Could you check a few things on this model? Use its own coordinates, in mm. Face numbers are marked on the shaded views. A direction names the side the tool comes from. Round coordinates to 2 decimals unless told otherwise and drop trailing zeros. Loops run counter-clockwise (first coordinate to the right, second up) from the corner with the lowest first, then second, coordinate; pieces in that order, holes last.
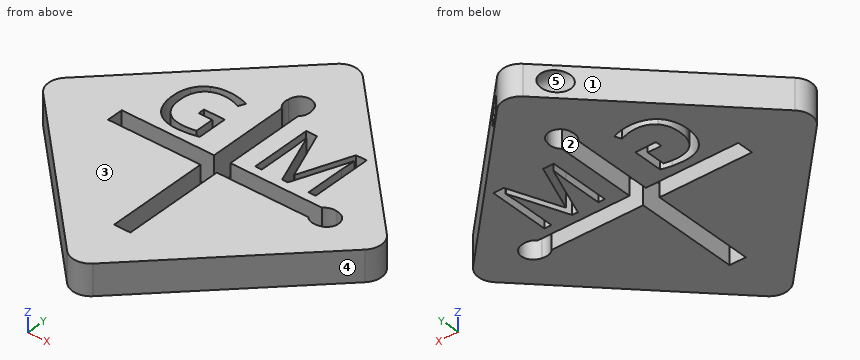
from build123d import *

# Parameters (mm, degrees)
F1_DEPTH = 2.5
F2_R     = 0.85
F3_DEPTH = 12.5


with BuildPart() as f1:
    # F0 (on Top) → F1 (new body)
    with BuildSketch(Plane.XY):
        with BuildLine():
            Line((13.081475452, -13.081475452), (1.0606601718, -1.0606601718))
            ThreePointArc((1.0606601718, -1.0606601718), (0, -0.6213203436), (-1.0606601718, -1.0606601718))
            Line((-1.0606601718, -1.0606601718), (-13.081475452, -13.081475452))
            ThreePointArc((-13.081475452, -13.081475452), (-13.5208152802, -14.1421356237), (-13.081475452, -15.2027957955))
            Line((-13.081475452, -15.2027957955), (-1.0606601718, -27.2236110757))
            ThreePointArc((-1.0606601718, -27.2236110757), (0, -27.6629509039), (1.0606601718, -27.2236110757))
            Line((1.0606601718, -27.2236110757), (13.081475452, -15.2027957955))
            ThreePointArc((13.081475452, -15.2027957955), (13.5208152802, -14.1421356237), (13.081475452, -13.081475452))
        make_face()
        with BuildLine():
            Line((-4.2551746457, -10.6432923429), (-4.2551746457, -10.1278843568))
            Line((-4.2551746457, -10.1278843568), (-2.5700617985, -10.1278843568))
            Line((-2.5700617985, -10.1278843568), (-2.5700617985, -12.5389086623))
            add(Edge.make_bspline(
                [(-2.5700617985, -12.5389086623), (-2.9639420069, -12.6647767179), (-3.3708430485, -12.7293383498)],
                knots=[0, 0, 0, 1, 1, 1], degree=2))
            add(Edge.make_bspline(
                [(-3.3708430485, -12.7293383498), (-3.7777440902, -12.7938999818), (-4.3137683957, -12.7938999818)],
                knots=[0, 0, 0, 1, 1, 1], degree=2))
            add(Edge.make_bspline(
                [(-4.3137683957, -12.7938999818), (-5.4389854096, -12.7938999818), (-6.0661555485, -12.1238695998)],
                knots=[0, 0, 0, 1, 1, 1], degree=2))
            add(Edge.make_bspline(
                [(-6.0661555485, -12.1238695998), (-6.6933256874, -11.4538392179), (-6.6933256874, -10.2472419957)],
                knots=[0, 0, 0, 1, 1, 1], degree=2))
            add(Edge.make_bspline(
                [(-6.6933256874, -10.2472419957), (-6.6933256874, -9.4735874818), (-6.3829958263, -8.8919902595)],
                knots=[0, 0, 0, 1, 1, 1], degree=2))
            add(Edge.make_bspline(
                [(-6.3829958263, -8.8919902595), (-6.0726659652, -8.3103930373), (-5.4894411388, -8.0038609193)],
                knots=[0, 0, 0, 1, 1, 1], degree=2))
            add(Edge.make_bspline(
                [(-5.4894411388, -8.0038609193), (-4.9062163124, -7.6973288012), (-4.123881243, -7.6973288012)],
                knots=[0, 0, 0, 1, 1, 1], degree=2))
            add(Edge.make_bspline(
                [(-4.123881243, -7.6973288012), (-3.3296104096, -7.6973288012), (-2.6449315902, -7.9881274123)],
                knots=[0, 0, 0, 1, 1, 1], degree=2))
            Line((-2.6449315902, -7.9881274123), (-2.8684558957, -8.4970249818))
            add(Edge.make_bspline(
                [(-2.8684558957, -8.4970249818), (-3.5401138819, -8.2127367873), (-4.1607736041, -8.2127367873)],
                knots=[0, 0, 0, 1, 1, 1], degree=2))
            add(Edge.make_bspline(
                [(-4.1607736041, -8.2127367873), (-5.0657215207, -8.2127367873), (-5.5746190902, -8.7514737665)],
                knots=[0, 0, 0, 1, 1, 1], degree=2))
            add(Edge.make_bspline(
                [(-5.5746190902, -8.7514737665), (-6.0835166596, -9.2902107457), (-6.0835166596, -10.2472419957)],
                knots=[0, 0, 0, 1, 1, 1], degree=2))
            add(Edge.make_bspline(
                [(-6.0835166596, -10.2472419957), (-6.0835166596, -11.2509312318), (-5.5936078055, -11.7695944262)],
                knots=[0, 0, 0, 1, 1, 1], degree=2))
            add(Edge.make_bspline(
                [(-5.5936078055, -11.7695944262), (-5.1036989513, -12.2882576207), (-4.1542631874, -12.2882576207)],
                knots=[0, 0, 0, 1, 1, 1], degree=2))
            add(Edge.make_bspline(
                [(-4.1542631874, -12.2882576207), (-3.6388552013, -12.2882576207), (-3.147318743, -12.1688999818)],
                knots=[0, 0, 0, 1, 1, 1], degree=2))
            Line((-3.147318743, -12.1688999818), (-3.147318743, -10.6432923429))
            Line((-3.147318743, -10.6432923429), (-4.2551746457, -10.6432923429))
        make_face(mode=Mode.SUBTRACT)
        with BuildLine():
            Line((-8.1334756687, -14.8039748892), (-8.1334756687, -13.4802963582))
            Line((-8.1334756687, -13.4802963582), (-0.6236797201, -13.4802963582))
            Line((-0.6236797201, -13.4802963582), (-0.6236797201, -6.9198086858))
            ThreePointArc((-0.6236797201, -6.9198086858), (-0.9032194318, -6.4583786209), (-0.9135835525, -5.9189782686))
            ThreePointArc((-0.9135835525, -5.9189782686), (0.0168397474, -5.0141534426), (0.9868078824, -5.876451129))
            ThreePointArc((0.9868078824, -5.876451129), (0.9900106564, -6.4384308628), (0.6999988109, -6.9198086858))
            Line((0.6999988109, -6.9198086858), (0.6999988109, -13.4802963582))
            Line((0.6999988109, -13.4802963582), (8.1334756687, -13.4802963582))
            ThreePointArc((8.1334756687, -13.4802963582), (8.5949057336, -13.2007566465), (9.134306086, -13.1903925258))
            ThreePointArc((9.134306086, -13.1903925258), (10.0391309119, -14.1208158258), (9.1768332255, -15.0907839607))
            ThreePointArc((9.1768332255, -15.0907839607), (8.6148534917, -15.0939867347), (8.1334756687, -14.8039748892))
            Line((8.1334756687, -14.8039748892), (0.6999988109, -14.8039748892))
            Line((0.6999988109, -14.8039748892), (0.6999988109, -23.1867600232))
            Line((0.6999988109, -23.1867600232), (-0.6236797201, -23.1867600232))
            Line((-0.6236797201, -23.1867600232), (-0.6236797201, -14.8039748892))
            Line((-0.6236797201, -14.8039748892), (-8.1334756687, -14.8039748892))
        make_face(mode=Mode.SUBTRACT)
        with BuildLine():
            Line((4.7664273717, -12.7628665604), (4.3020176494, -12.7628665604))
            Line((4.3020176494, -12.7628665604), (2.6201600105, -8.3683353104))
            Line((2.6201600105, -8.3683353104), (2.5930332744, -8.3683353104))
            add(Edge.make_bspline(
                [(2.5930332744, -8.3683353104), (2.64077633, -8.8902537131), (2.64077633, -9.6096547548)],
                knots=[0, 0, 0, 1, 1, 1], degree=2))
            Line((2.64077633, -9.6096547548), (2.64077633, -12.7628665604))
            Line((2.64077633, -12.7628665604), (2.1080072328, -12.7628665604))
            Line((2.1080072328, -12.7628665604), (2.1080072328, -7.8051842687))
            Line((2.1080072328, -7.8051842687), (2.9760627883, -7.8051842687))
            Line((2.9760627883, -7.8051842687), (4.5461582744, -11.8948110048))
            Line((4.5461582744, -11.8948110048), (4.5732850105, -11.8948110048))
            Line((4.5732850105, -11.8948110048), (6.15640133, -7.8051842687))
            Line((6.15640133, -7.8051842687), (7.0179464689, -7.8051842687))
            Line((7.0179464689, -7.8051842687), (7.0179464689, -12.7628665604))
            Line((7.0179464689, -12.7628665604), (6.4417745939, -12.7628665604))
            Line((6.4417745939, -12.7628665604), (6.4417745939, -9.5684221159))
            add(Edge.make_bspline(
                [(6.4417745939, -9.5684221159), (6.4417745939, -9.019376977), (6.4895176494, -8.374845727)],
                knots=[0, 0, 0, 1, 1, 1], degree=2))
            Line((6.4895176494, -8.374845727), (6.4623909133, -8.374845727))
            Line((6.4623909133, -8.374845727), (4.7664273717, -12.7628665604))
        make_face(mode=Mode.SUBTRACT)
    extrude(amount=F1_DEPTH)

    # F2 (on Right) → F3 (cut, symmetric)
    with BuildSketch(Plane.YZ):
        with Locations((-2.4908210296, 1.292226194)):
            Circle(F2_R)
    extrude(amount=F3_DEPTH, both=True, mode=Mode.SUBTRACT)


solid = f1.part
Item 1: If we section it at D-D, the plane x = -11: Please give me the cut outline in (y, z), then the cut area to 3 significant figures.
Results list:
outline: (-17.28, 0) - (-11, 0) - (-11, 2.5) - (-17.28, 2.5) - close
area: 15.7 mm2
Item 2: Will these pins go through, and if not, where does the flat tip stop? pin 1 (0.8 mm diameter, centred on y = -9.5, z = 1, fed in from -X); pin 2 (1.2 mm diameter, centred on x = 5.5, z = 1, fed in from +Y); pin 3 (12 mm diameter, centred on x = -9, y = -19.5, fed in from +Z); pin 4 (1.2 mm diameter, centred on y = -20, z = 1.5, fed in from +X).
Results list:
pin 1: stops at x = -9.9
pin 2: stops at y = -4.9
pin 3: stops at z = 2.5
pin 4: stops at x = 8.88
Item 3: We'd pull the mould along Z, two halves only. Please class the marked faces 3, 4 and 5: released by +Z, released by -Z, zero draft, split by the parting line, or undercut.
Results list:
face 3: released by +Z
face 4: zero draft
face 5: undercut
Item 4: If we section it at B-B, the plane x = -7.75: Please give me the cut outline in (y, z), then the cut area to 3 significant figures.
Results list:
outline: (-20.53, 0) - (-14.8, 0) - (-14.8, 2.5) - (-20.53, 2.5) - close; (-13.48, 0) - (-7.75, 0) - (-7.75, 2.5) - (-13.48, 2.5) - close
area: 28.7 mm2
Item 5: If we section it at A-A, the plane y = -18.75: Please give me the cut outline in (x, z), then the cut area to 3 significant figures.
Results list:
outline: (-9.53, 0) - (-0.62, 0) - (-0.62, 2.5) - (-9.53, 2.5) - close; (0.7, 0) - (9.53, 0) - (9.53, 2.5) - (0.7, 2.5) - close
area: 44.4 mm2
Item 6: For the marked faces 1 and 2, which set-ups out of +Z, -Z, +X, -X, +Y, -Y let a thin tool reach every point of the face, with its end or its side?
Results list:
face 1: +Z, -Z, -X, +Y
face 2: +Z, -Z
Item 7: If we section it at C-C, the plane z = 0.9: Count the separate pieces of the cut face and the enclosed holes in it, then the cut area to 3 significant figures.
Results list:
separate pieces: 2
enclosed holes: 3
area: 325 mm2
Item 8: If I drill on line 1 along Y through (x, z) = (0.75, 1.45); line 2 along Y through (x, z) = (-0.25, 1.8); line 3 along X through (y, z) = (-12.5, 0.35), over which ranges is the centre line in solid material (lowest first)?
Results list:
line 1: y = -27.46 to -14.8, -13.48 to -6.87, -5.33 to -3.33, -1.66 to -0.82
line 2: y = -27.64 to -23.19, -5.06 to -3.17, -1.81 to -0.64
line 3: x = -12.5 to -5.59, -2.57 to -0.62, 0.7 to 2.11, 2.64 to 4.2, 4.87 to 6.44, 7.02 to 12.5
